Read the model definition and answer for the solid it produces. Units are mm, in the model's axes. A direction names the side the tool comes from. Coordinates: 2 decimals unless noted, no trailing zeros. Order: outer loops, then holes, each group sorted by start corner. A loop starts at its lowest first (then second) coordinate and runs counter-clockwise, first axis right, second up. Notation, with made-up numbers: (82, 20.5) - (93, 20.5) arc R15 ccw to (93, 33.5) - close; hole circle Ø1 at (66.25, 78). An arc over 180 degrees is marked (long way). Write item = value, one per line.
Autodesk Fusion 360 part; units mm, degrees
sketch "Sketch3" plane through (0, 0, 0) normal (0, 0, 1) x (1, 0, 0)
  line L0 (12.2, 7.0437) -> (0, 14.0873)
  line L1 (0, 14.0873) -> (-12.2, 7.0437)
  line L2 (-12.2, 7.0437) -> (-12.2, -7.0437)
  line L3 (-12.2, -7.0437) -> (0, -14.0873)
  line L4 (0, -14.0873) -> (12.2, -7.0437)
  line L5 (12.2, -7.0437) -> (12.2, 7.0437)
  line L6 (0, -14.0873) -> (0, 14.0873) construction
  line L7 (24.4, 14.0873) -> (24.4, 28.1747)
  line L8 (24.4, 28.1747) -> (12.2, 35.2184)
  line L9 (12.2, 35.2184) -> (0, 28.1747)
  line L10 (0, 28.1747) -> (0, 14.0873)
  line L11 (0, 14.0873) -> (12.2, 7.0437)
  line L12 (12.2, 7.0437) -> (24.4, 14.0873)
  line L13 (0, 14.0873) -> (0, 28.1747)
  line L14 (0, 28.1747) -> (-12.2, 35.2184)
  line L15 (-12.2, 35.2184) -> (-24.4, 28.1747)
  line L16 (-24.4, 28.1747) -> (-24.4, 14.0873)
  line L17 (-24.4, 14.0873) -> (-12.2, 7.0437)
  line L18 (-12.2, 7.0437) -> (0, 14.0873)
  line L19 (36.6, -7.0437) -> (36.6, 7.0437)
  line L20 (36.6, 7.0437) -> (24.4, 14.0873)
  line L21 (24.4, 14.0873) -> (12.2, 7.0437)
  line L22 (12.2, 7.0437) -> (12.2, -7.0437)
  line L23 (12.2, -7.0437) -> (24.4, -14.0873)
  line L24 (24.4, -14.0873) -> (36.6, -7.0437)
  line L25 (-12.2, 7.0437) -> (-24.4, 14.0873)
  line L26 (-24.4, 14.0873) -> (-36.6, 7.0437)
  line L27 (-36.6, 7.0437) -> (-36.6, -7.0437)
  line L28 (-36.6, -7.0437) -> (-24.4, -14.0873)
  line L29 (-24.4, -14.0873) -> (-12.2, -7.0437)
  line L30 (-12.2, -7.0437) -> (-12.2, 7.0437)
  line L31 (-12.2, -7.0437) -> (-24.4, -14.0873)
  line L32 (-24.4, -14.0873) -> (-24.4, -28.1747)
  line L33 (-24.4, -28.1747) -> (-12.2, -35.2184)
  line L34 (-12.2, -35.2184) -> (0, -28.1747)
  line L35 (0, -28.1747) -> (0, -14.0873)
  line L36 (0, -14.0873) -> (-12.2, -7.0437)
  line L37 (24.4, -14.0873) -> (12.2, -7.0437)
  line L38 (12.2, -7.0437) -> (0, -14.0873)
  line L39 (0, -14.0873) -> (0, -28.1747)
  line L40 (0, -28.1747) -> (12.2, -35.2184)
  line L41 (12.2, -35.2184) -> (24.4, -28.1747)
  line L42 (24.4, -28.1747) -> (24.4, -14.0873)
  line L43 (0, 48) -> (0, -40) construction
  point P0 (12.2, 21.131)
  point P1 (-12.2, 21.131)
  point P2 (24.4, 0)
  point P3 (-24.4, 0)
  point P4 (-12.2, -21.131)
  point P5 (12.2, -21.131)
  dimension "d10" = 12.2
  dimension "d29" = 12.2
  dimension "d30" = 12.2
  dimension "d31" = 12.2
  dimension "d32" = 12.2
  dimension "d33" = 12.2
  dimension "d34" = 12.2
extrude "Extrude2" add sketch "Sketch3" along normal blind 3
sketch "Sketch4" plane through (0, 0, 3) normal (0, 0, 1) x (1, 0, 0)
  line L0 (13.5653, 29.6958) -> (-18.9347, -26.5958)
  line L1 (-18.9347, -26.5958) -> (-17.2026, -27.5958)
  line L2 (-17.2026, -27.5958) -> (15.2974, 28.6958)
  line L3 (15.2974, 28.6958) -> (13.5653, 29.6958)
  line L4 (17.2026, 27.5958) -> (-15.2974, -28.6958)
  line L5 (-15.2974, -28.6958) -> (-13.5653, -29.6958)
  line L6 (-13.5653, -29.6958) -> (18.9347, 26.5958)
  line L7 (18.9347, 26.5958) -> (17.2026, 27.5958)
  line L8 (-24.4, 14.0873) -> (24.4, -14.0873) construction
  line L9 (24.4, -28.1747) -> (24.4, -14.0873)
  line L10 (24.4, -14.0873) -> (36.6, -7.0437)
  line L11 (36.6, -7.0437) -> (36.6, 7.0437)
  line L12 (36.6, 7.0437) -> (24.4, 14.0873)
  line L13 (24.4, 14.0873) -> (24.4, 28.1747)
  line L14 (24.4, 28.1747) -> (12.2, 35.2184)
  line L15 (12.2, 35.2184) -> (0, 28.1747)
  line L16 (0, 28.1747) -> (-12.2, 35.2184)
  line L17 (-12.2, 35.2184) -> (-24.4, 28.1747)
  line L18 (-24.4, 28.1747) -> (-24.4, 14.0873)
  line L19 (-24.4, 14.0873) -> (-36.6, 7.0437)
  line L20 (-36.6, 7.0437) -> (-36.6, -7.0437)
  line L21 (-36.6, -7.0437) -> (-24.4, -14.0873)
  line L22 (-24.4, -14.0873) -> (-24.4, -28.1747)
  line L23 (-24.4, -28.1747) -> (-12.2, -35.2184)
  line L24 (-12.2, -35.2184) -> (0, -28.1747)
  line L25 (0, -28.1747) -> (12.2, -35.2184)
  line L26 (12.2, -35.2184) -> (24.4, -28.1747)
  line L27 (18.3, 31.6965) -> (-18.3, -31.6965)
  dimension "d13" = 65
  dimension "d14" = 2
  dimension "d15" = 2.2
extrude "Extrude3" add sketch "Sketch4" along normal blind 7 contours L0 L1 L2 L3 | L4 L5 L6 L7
sketch "Sketch5" plane through (0, 0, 0) normal (0, 0, -1) x (-1, 0, 0)
  line L0 (-17.2026, 27.5958) -> (-15.2974, 28.6958)
  line L1 (-15.2974, 28.6958) -> (17.2026, -27.5958)
  line L2 (17.2026, -27.5958) -> (15.2974, -28.6958)
  line L3 (15.2974, -28.6958) -> (-17.2026, 27.5958)
  line L4 (24.4, -28.1747) -> (12.2, -35.2184)
  line L5 (-24.4, 28.1747) -> (-12.2, 35.2184)
  line L6 (18.3, -31.6965) -> (-18.3, 31.6965) construction
  line L7 (24.4, 14.0873) -> (-24.4, -14.0873) construction
  line L8 (24.4, 14.0873) -> (36.6, 7.0437)
  point P0 (24.4, 14.0873)
  point P1 (-24.4, -14.0873)
  dimension "d18" = 65
  dimension "d19" = 2.2
extrude "Extrude4" cut sketch "Sketch5" against normal blind 2
fillet "Fillet1" radius 4 4 edges at (-14.4313, -29.1958, 10) (-18.0687, -27.0958, 10) (18.0687, 27.0958, 10) (14.4313, 29.1958, 10)
fillet "Fillet2" radius 2 12 edges at (-12.2, -35.2184, 1.5) (12.2, -35.2184, 1.5) (24.4, -28.1747, 1.5) (36.6, -7.0437, 1.5) (36.6, 7.0437, 1.5) (24.4, 28.1747, 1.5) (12.2, 35.2184, 1.5) (-12.2, 35.2184, 1.5) (-24.4, 28.1747, 1.5) (-36.6, 7.0437, 1.5) (-36.6, -7.0437, 1.5) (-24.4, -28.1747, 1.5)
fillet "Fillet3" radius 0.5 4 edges at (-16.25, -28.1458, 0) (-0.9526, 0.55, 0) (16.25, 28.1458, 0) (0.9526, -0.55, 0)
fillet "Fillet5" radius 2 30 edges at (-5.6, 31.4079, 3) (-12.2, 34.909, 3) (-18.3, 31.6965, 3) (-24.1321, 28.02, 3) (-24.4, 20.5537, 3) (24.4, 20.5537, 3) (24.1321, 28.02, 3) (18.3, 31.6965, 3) (12.2, 34.909, 3) (5.6, 31.4079, 3) (30, -10.8542, 3) (36.3321, -6.889, 3) (36.6, 0, 3) (36.3321, 6.889, 3) (30, 10.8542, 3) (5.6, -31.4079, 3) (12.2, -34.909, 3) (18.3, -31.6965, 3) (24.1321, -28.02, 3) (24.4, -20.5537, 3) (-24.4, -20.5537, 3) (-24.1321, -28.02, 3) (-18.3, -31.6965, 3) (-12.2, -34.909, 3) (-5.6, -31.4079, 3) (-30, 10.8542, 3) (-36.3321, 6.889, 3) (-36.6, 0, 3) (-36.3321, -6.889, 3) (-30, -10.8542, 3)
1) Determine the mould class of faces 6 (the face through (29.3, -10.6, 2.4)), 7 (the face through (-18.229, 31.738, 0.493)), 8 (the face through (-5.49, 30.65, 2.43)), 9 (the face through (8, 0, 0)) for opening direction X: pulls with the +X half, pulls with the -X half, needs draft (parallel to the pull), parting line crosses it, or undercut.
Returned:
face_6 = pulls with the +X half
face_7 = pulls with the -X half
face_8 = undercut
face_9 = needs draft
2) Straight lines are drawn through the part: line 1 along X through (y, z) = (-21.5, 4.75); line 2 along X through (y, z) = (18.5, 1); line 3 along Y through (x, z) = (14.5, 6.75). For each, find the intervals that lie inside material, in ascending order. Write a range as from..to.
Returned:
line_1 = -15.99..-13.68, -11.14..-8.83
line_2 = -24.4..9.41, 11.95..24.4
line_3 = 18.91..22.91, 27.31..29.07
3) For faces 1 (the face through (-1.314, 0.225, 0.143)), 2 (the face through (-18.08, -27.09, 4.48)), 3 (the face through (14.44, 29.19, 4.48)), 4 (the face through (-5.678, -31.453, 0.493)), 5 (the face through (-5.52, 31.36, 0.49)), determine the directions among +Z, -Z, +X, -X, +Y, -Y from which every point of the face is accessible in a straight line to the end or side of a thin tool.
Returned:
face_1 = -Z
face_2 = +Z, -X, -Y
face_3 = +Z, +X, +Y
face_4 = +Z, -Z, -Y
face_5 = +Z, -Z, +Y
4) The part is cut by section A-A (z = 7.25). Determine the outline of the cut face in (x, y), and give its area (3 significant figures).
Returned:
outline = (-18.83, -26.42) - (-17.1, -27.42) - (15.2, 28.52) - (13.47, 29.52) - close; (-15.2, -28.52) - (-13.47, -29.52) - (18.83, 26.42) - (17.1, 27.42) - close
area = 258 mm^2
5) Flat-ended cylindrical pins translate along their axes: pin 1 Ø1.5 at (x, y) = (14.5, -23.5) entering from +Z; pin 2 Ø12 at (x, y) = (-7.5, 19.5) entering from -Z; pin 3 Ø1.1 at (y, z) = (-22, 0.5) entering from +X; pin 4 Ø2 at (y, z) = (22, 9) entering from -X. Find the tip coordinate at first contact, or state that the pin passes through.
Returned:
pin_1 = 3
pin_2 = 0
pin_3 = 24.4
pin_4 = 8.54
